For this review, take the finished solid that the model builds, in its own axes (mm). A direction names the side the tool comes from. Give positions to 0.01 mm unless a question says otherwise; leave off trailing zeros. Order: outer loops, then holes, each group sorted by start corner. A loop starts at its lowest first (then second) coordinate and runs counter-clockwise, first axis right, second up.
from build123d import *

# Parameters (mm, degrees)
F0_W          = 31.75
F0_H          = 72.39
F1_DEPTH      = 38.1
F1_DEPTH_BACK = 38.1
F2_R          = 8.255
F2_R_2        = 4.28625
F3_DEPTH      = 6.35
F3_FACE_R     = 4.28625
F4_DEPTH      = 72.391


with BuildPart() as f1:
    # F0 (on Right) → F1 (new body, two sides)
    with BuildSketch(Plane.YZ) as f1_sk:
        Rectangle(F0_W, F0_H)
    extrude(amount=F1_DEPTH)
    extrude(f1_sk.sketch, amount=-F1_DEPTH_BACK)

    # F2 (on face) → F3 (cut)
    with BuildSketch(Plane.XY.offset(36.195)):
        Circle(F2_R)
        Circle(F2_R_2, mode=Mode.SUBTRACT)
    extrude(amount=-F3_DEPTH, mode=Mode.SUBTRACT)

    # F3_face (on face) → F4 (cut, through all)
    with BuildSketch(Plane.XY.offset(36.195)):
        Circle(F3_FACE_R)
    extrude(amount=-F4_DEPTH, mode=Mode.SUBTRACT)


solid = f1.part
1) To check wall thickness, follow line 1 (Y direction, x = 0, z = -18) (3 decimals); line 2 (Y direction, x = 0, z = 32.5) (3 decimals); line 3 (X direction, y = 3.5, z = 3). State the ranges of each line that lie inside material, in increasing order.
Answer sheet:
line 1: y = -15.875 to -4.286, 4.286 to 15.875
line 2: y = -15.875 to -8.255, 8.255 to 15.875
line 3: x = -38.1 to -2.47, 2.47 to 38.1
2) We need section A-A on y = 0. Give the boundary of the cut face in (x, z) (3 decimals), then the cut area to 3 significant figures.
Answer sheet:
outline: (-38.1, -36.195) - (-4.286, -36.195) - (-4.286, 29.845) - (-8.255, 29.845) - (-8.255, 36.195) - (-38.1, 36.195) - close; (4.286, -36.195) - (38.1, -36.195) - (38.1, 36.195) - (8.255, 36.195) - (8.255, 29.845) - (4.286, 29.845) - close
area: 4,850 mm2
3) Tool access review of faces 4 (the face through (-38.1, 0, 1)), 5 (the face through (4, -4, 29.845)): name each direction out of +Z, -Z, +X, -X, +Y, -Y from which nothing blocks a thin tool from reaching the whole face with its end or side.
Answer sheet:
face 4: +Z, -Z, -X, +Y, -Y
face 5: +Z
4) We need section B-B on x = 0. Give the boundary of the cut face in (y, z) (3 decimals).
Answer sheet:
outline: (-15.875, -36.195) - (-4.286, -36.195) - (-4.286, 29.845) - (-8.255, 29.845) - (-8.255, 36.195) - (-15.875, 36.195) - close; (4.286, -36.195) - (15.875, -36.195) - (15.875, 36.195) - (8.255, 36.195) - (8.255, 29.845) - (4.286, 29.845) - close
5) We need section C-C on z = -6. Give the boundary of the cut face in (x, y) (1 decimal), then the cut area to 3 significant figures.
Answer sheet:
outline: (-38.1, -15.9) - (38.1, -15.9) - (38.1, 15.9) - (-38.1, 15.9) - close; hole circle Ø8.6 at (0, 0)
area: 2,360 mm2
6) Draft analysis for pull direction Y (two halves, no side actions). For faces 1 (the face through (1, 7, -36.195)), 2 (the face through (2.304, 3.614, -2.713)), 3 (the face through (1, -15.875, -1)), state which applies: +Y half, -Y half, draft (parallel to the pull), parting line (faces both ways), or undercut.
Answer sheet:
face 1: draft
face 2: undercut
face 3: -Y half
7) Clearance check with flat-ended pins moving along their axes: pin 1 (7.5 mm diameter, centred on x = 0, y = 0, fed in from -Z); pin 2 (8.5 mm diameter, centred on x = -2.5, y = -2.5, fed in from +Z) (3 decimals); pin 3 (19 mm diameter, centred on x = 0, y = 0, fed in from +Z) (3 decimals). State where each tip first meets the part, or that it passes through.
Answer sheet:
pin 1: passes through
pin 2: stops at z = 29.845
pin 3: stops at z = 36.195
